from build123d import *

# Parameters (mm, degrees)
F0_R     = 70.05
F1_DEPTH = 2
F2_R     = 1
F3_R     = 70.05
F3_R_2   = 69.55
F4_DEPTH = 1
F5_R     = 10
F6_DEPTH = 0.5
F7_R     = 3
F8_DEPTH = 1.5


with BuildPart() as f1:
    # F0 (on Top) → F1 (new body)
    with BuildSketch(Plane.XY):
        Circle(F0_R)
    extrude(amount=F1_DEPTH)

    # F2
    f2_edges = [f1.edges().sort_by_distance(p)[0] for p in [
        (-70.05, 0, 2),
    ]]
    fillet(f2_edges, radius=F2_R)

    # F3 (on face) → F4 (join)
    with BuildSketch(Plane(origin=(0, 0, 0), x_dir=(1, 0, 0), z_dir=(0, 0, -1))):
        Circle(F3_R)
        Circle(F3_R_2, mode=Mode.SUBTRACT)
    extrude(amount=F4_DEPTH)

    # F5 (on face) → F6 (cut)
    with BuildSketch(Plane.XY.offset(2)):
        Circle(F5_R)
    extrude(amount=-F6_DEPTH, mode=Mode.SUBTRACT)

    # F7 (on face) → F8 (cut, through all)
    with BuildSketch(Plane.XY.offset(1.5)):
        Circle(F7_R)
    extrude(amount=-F8_DEPTH, mode=Mode.SUBTRACT)


solid = f1.part
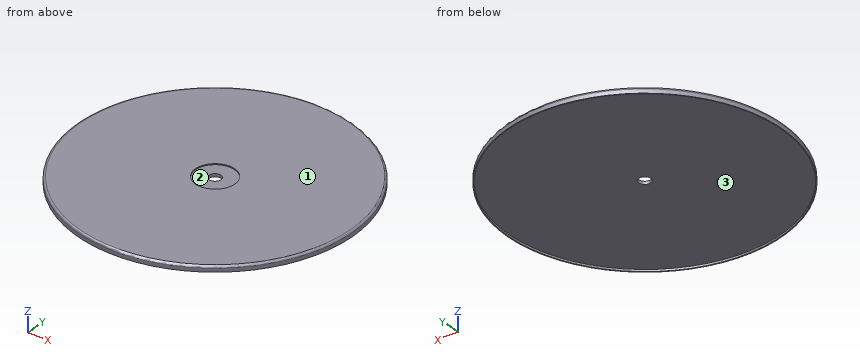
Can you work these out from the model? Positions are in its coordinate system, mm. Face numbers are marked on the shaded views. Give positions to 0.01 mm unless a question says otherwise; leave off trailing zeros. Order: outer loops, then holes, each group sorted by start corner. A loop starts at its lowest first (then second) coordinate and runs counter-clockwise, first axis right, second up. Notation, with made-up numbers: M -22,-15 L 8,-15 A28 cw 8,4 Z; hole C 5.5,52 d8. An arc over 180 degrees is marked long. One line per question, with ' | ' between items.
Item 1: We'd pull the mould along Y, two halves only. Please class the marked faces 1, 2 and 3: released by +Y, released by -Y, zero draft, split by the parting line, or undercut.
Answer block:
face 1: zero draft | face 2: undercut | face 3: undercut
Item 2: Suppose I cut it at A-A, the plane x = 0. Write out the boundary of the cut face in (y, z), then the cut area to 3 significant figures.
Answer block:
outline: M -70.05,-1 L -69.55,-1 L -69.55,0 L -3,0 L -3,1.5 L -10,1.5 L -10,2 L -69.05,2 A1 ccw -70.05,1 Z; M 3,0 L 69.55,0 L 69.55,-1 L 70.05,-1 L 70.05,1 A1 ccw 69.05,2 L 10,2 L 10,1.5 L 3,1.5 Z | area: 262 mm2
Item 3: I'm going to push flat-ended pins straight in: pin 1 Ø7 at (x, y) = (0, 0) entering from -Z; pin 2 Ø16 at (x, y) = (0, 0) entering from +Z. Where does each tip first touch, or does it pass through?
Answer block:
pin 1: stops at z = 0 | pin 2: stops at z = 1.5
Item 4: Please list where these lines run through material, in increasing order: L1, parallel to Y at x = 0, z = -0.15; L2, parallel to Y at x = 0, z = 0.55.
Answer block:
L1: y = -70.05 to -69.55, 69.55 to 70.05 | L2: y = -70.05 to -3, 3 to 70.05
